```python
from build123d import *

# Parameters (mm, degrees)
SKETCH1_W           = 40
SKETCH1_H           = 86
BOSS_EXTRUDE1_DEPTH = 12
SKETCH2_W           = 12
SKETCH2_H           = 86
BOSS_EXTRUDE2_DEPTH = 87
SKETCH3_R           = 3
CUT_EXTRUDE1_DEPTH  = 13
SKETCH4_R           = 38
CUT_EXTRUDE2_DEPTH  = 3
SKETCH5_R           = 2.6
CUT_EXTRUDE3_DEPTH  = 13
FILLET1_R           = 3
SKETCH6_R           = 20
CUT_EXTRUDE4_DEPTH  = 13
SKETCH7_W           = 40
SKETCH7_H           = 12
CUT_EXTRUDE5_DEPTH  = 87
FILLET2_R           = 1
SKETCH8_R           = 2.1
CUT_EXTRUDE6_DEPTH  = 12


with BuildPart() as part:
    # Sketch1 → Boss-Extrude1 (new body)
    with BuildSketch(Plane(origin=(0, 0, 0), x_dir=(1, 0, 0), z_dir=(0, 1, 0))):
        with Locations((20, -43)):
            Rectangle(SKETCH1_W, SKETCH1_H)
    extrude(amount=BOSS_EXTRUDE1_DEPTH)

    # Sketch2 → Boss-Extrude2 (add)
    with BuildSketch(Plane(origin=(0, 12, 0), x_dir=(1, 0, 0), z_dir=(0, 1, 0))):
        with Locations((34, -43)):
            Rectangle(SKETCH2_W, SKETCH2_H)
    extrude(amount=BOSS_EXTRUDE2_DEPTH)

    # Sketch3 → Cut-Extrude1 (cut, through all)
    with BuildSketch(Plane(origin=(0, 12, 0), x_dir=(1, 0, 0), z_dir=(0, 1, 0))):
        with Locations((14, -8.4)):
            Circle(SKETCH3_R)
        with Locations((14, -77.6)):
            Circle(SKETCH3_R)
    extrude(amount=-CUT_EXTRUDE1_DEPTH, mode=Mode.SUBTRACT)

    # Sketch4 → Cut-Extrude2 (cut)
    with BuildSketch(Plane.ZY.offset(-28)):
        with Locations((43, 56)):
            Circle(SKETCH4_R)
    extrude(amount=-CUT_EXTRUDE2_DEPTH, mode=Mode.SUBTRACT)

    # Sketch5 → Cut-Extrude3 (cut, through all)
    with BuildSketch(Plane.ZY.offset(-28)):
        with Locations((77.8, 90.8)):
            Circle(SKETCH5_R)
        with Locations((77.8, 21.2)):
            Circle(SKETCH5_R)
        with Locations((8.2, 90.8)):
            Circle(SKETCH5_R)
        with Locations((8.2, 21.2)):
            Circle(SKETCH5_R)
    extrude(amount=-CUT_EXTRUDE3_DEPTH, mode=Mode.SUBTRACT)

    # Fillet1
    fillet1_edges = [part.edges().sort_by_distance(p)[0] for p in [
        (34, 99, 0),
        (34, 99, 86),
    ]]
    fillet(fillet1_edges, radius=FILLET1_R)

    # Sketch6 → Cut-Extrude4 (cut, through all)
    with BuildSketch(Plane.ZY.offset(-28)):
        with Locations((43, 56)):
            Circle(SKETCH6_R)
    extrude(amount=-CUT_EXTRUDE4_DEPTH, mode=Mode.SUBTRACT)

    # Sketch7 → Cut-Extrude5 (cut, through all)
    with BuildSketch(Plane.XY.offset(86)):
        with Locations((20, 6)):
            Rectangle(SKETCH7_W, SKETCH7_H)
    extrude(amount=-CUT_EXTRUDE5_DEPTH, mode=Mode.SUBTRACT)

    # Fillet2
    fillet2_edges = [part.edges().sort_by_distance(p)[0] for p in [
        (34, 12, 0),
        (34, 12, 86),
    ]]
    fillet(fillet2_edges, radius=FILLET2_R)

    # Sketch8 → Cut-Extrude6 (cut)
    with BuildSketch(Plane.XZ.offset(-12)):
        with Locations((34, 70)):
            Circle(SKETCH8_R)
        with Locations((34, 16)):
            Circle(SKETCH8_R)
    extrude(amount=-CUT_EXTRUDE6_DEPTH, mode=Mode.SUBTRACT)


solid = part.part
```
The model under review builds one solid part; all positions refer to its coordinate system, in mm. A direction names the side the tool comes from. Coordinates: 2 decimals unless noted, no trailing zeros. Write each loop counter-clockwise with the first axis right and the second up, starting at its lowest first coordinate (ties: lowest second). Pieces come first, ordered by that corner, then holes. Notation, with made-up numbers: (-22.75, 66) - (-14.75, 66) arc R26 ccw to (-14.75, 94) - close; hole circle Ø1 at (-25.5, 66). An arc over 180 degrees is marked (long way). Answer in a Markdown table with one row per item. Add a question column.
Q1. Draft analysis for pull direction Y (two halves, no side actions). For faces 1 (the face through (29.479, 67.414, 79.245)), 2 (the face through (34.08, 98.1, 85.14)), 3 (the face through (34, 24, 70)), state which applies: +Y half, -Y half, draft (parallel to the pull), parting line (faces both ways), or undercut.
Q2. Consider section D-D on y = 21.2. Give the boundary of the cut face in (x, z), then the cut area to 3 significant figures.
Q3. Consider section A-A on x = 34. Give the boundary of the cut face in (y, z).
Q4. For faces 4 (the face through (33.9, 20.2, 80.2)), 5 (the face through (32.334, 17.916, 68.722)), 6 (the face through (31, 40, 59)), list the 3-axis set-ups (+Z, -Z, +X, -X, +Y, -Y) from which the entire face can be reached by the end or side of a thin tool; tool diameter is ignored.
Q5. To check wall thickness, follow line 1 along Y through (x, z) = (37, 8.2); line 2 along Z through (x, y) = (34, 15); line 3 along Y through (x, z) = (39, 77). State the ranges of each line that lie inside material, in increasing order. Write a range as from..to.
Q6. Consider section C-C on y = 56. Give the boundary of the cut face in (x, z), then the cut area to 3 significant figures.
Q7. Consider section B-B on z = 43. Give the boundary of the cut face in (x, y), then the cut area to 3 significant figures.
Q8. Clearance check with flat-ended pins moving along their axes: pin 1 (1.5 mm diameter, centred on y = 30.5, z = 43.5, fed in from -X); pin 2 (4 mm diameter, centred on x = 34, z = 16, fed in from -Y). State where each tip first meets the part, or that it passes through.
Answers below:
| question | item | result |
|---|---|---|
| 1 | face 1 | undercut |
| 1 | face 2 | +Y half |
| 1 | face 3 | -Y half |
| 2 | outline | (28, 0) - (40, 0) - (40, 5.6) - (28, 5.6) - close; (28, 10.8) - (40, 10.8) - (40, 75.2) - (28, 75.2) - (28, 58.26) - (31, 58.26) - (31, 27.74) - (28, 27.74) - close; (28, 80.4) - (40, 80.4) - (40, 86) - (28, 86) - close; hole circle Ø4.2 at (34, 16); hole circle Ø4.2 at (34, 70) |
| 2 | area | 788 mm² |
| 3 | outline | (12, 1) arc R1 ccw to (13, 0) - (96, 0) arc R3 ccw to (99, 3) - (99, 83) arc R3 ccw to (96, 86) - (13, 86) arc R1 ccw to (12, 85) - (12, 72.1) - (24, 72.1) - (24, 67.9) - (12, 67.9) - (12, 18.1) - (24, 18.1) - (24, 13.9) - (12, 13.9) - close; hole circle Ø5.2 at (21.2, 8.2); hole circle Ø5.2 at (21.2, 77.8); hole circle Ø40 at (56, 43); hole circle Ø5.2 at (90.8, 8.2); hole circle Ø5.2 at (90.8, 77.8) |
| 4 | face 4 | +X, -X |
| 4 | face 5 | -Y |
| 4 | face 6 | -X |
| 5 | line 1 | 12..18.6, 23.8..88.2, 93.4..99 |
| 5 | line 2 | 0..13.9, 18.1..67.9, 72.1..86 |
| 5 | line 3 | 12..18.73, 23.67..88.33, 93.27..99 |
| 6 | outline | (28, 0) - (40, 0) - (40, 23) - (31, 23) - (31, 5) - (28, 5) - close; (28, 81) - (31, 81) - (31, 63) - (40, 63) - (40, 86) - (28, 86) - close |
| 6 | area | 444 mm² |
| 7 | outline | (28, 12) - (40, 12) - (40, 36) - (31, 36) - (31, 18) - (28, 18) - close; (28, 94) - (31, 94) - (31, 76) - (40, 76) - (40, 99) - (28, 99) - close |
| 7 | area | 456 mm² |
| 8 | pin 1 | x = 31 |
| 8 | pin 2 | y = 24 |
